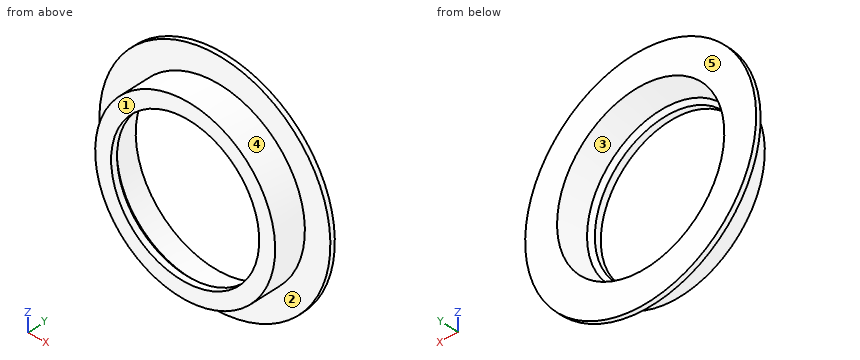
```python
from build123d import *

# Parameters (mm, degrees)
CHAMFER1_SIZE2 = 1
CHAMFER1_SIZE  = 1.294432523


with BuildPart() as part:
    # Sketch2 → Revolve1 (revolve)
    with BuildSketch(Plane.XY, mode=Mode.PRIVATE) as revolve1_sk:
        Polygon((28.25, 0), (28.25, 10), (36.25, 10), (36.25, 11.5), (26.25, 11.5), (24.25, 2), (23.25, 2), (23.25, 0), align=None)
    revolve(revolve1_sk.sketch.rotate(Axis((0, 0, 0), (0, 1, 0)), 90), axis=Axis((0, 0, 0), (0, 1, 0)))

    # Chamfer1
    chamfer1_edges = [part.edges().sort_by_distance(p)[0] for p in [
        (0, 2, 24.25),
    ]]
    chamfer1_side = [part.faces().sort_by_distance(p)[0] for p in [
        (0, 2.019570996, 24.25412021),
    ]]
    chamfer(chamfer1_edges, length=CHAMFER1_SIZE - 0.0001, length2=CHAMFER1_SIZE2 - 0.0001, reference=chamfer1_side[0])  # a hair under: the kernel refuses the full size


solid = part.part
```
For this review, take the finished solid that the model builds, in its own axes (mm). Face numbers are marked on the shaded views. A direction names the side the tool comes from. Coordinates: 2 decimals unless noted, no trailing zeros. Write each loop counter-clockwise with the first axis right and the second up, starting at its lowest first coordinate (ties: lowest second). Pieces come first, ordered by that corner, then holes. Notation, with made-up numbers: (79, -32.75) -> (99, -32.75) arc R12 cw to (99, -18.75) -> close; hole circle Ø10 at (81, 66). An arc over 180 degrees is marked (long way). Put each result on its own line as item: value.
Q1. Take a section at D-D, the plane y = 7. State the section outline as (x, z) points, then the cut area to 3 significant figures.
From the geometry:
outline: circle Ø56.5 at (0, 0); hole circle Ø50.61 at (0, 0)
area: 496 mm2
Q2. Clearance check with flat-ended pins moving along their axes: pin 1 Ø6 at (y, z) = (9, 11.5) entering from -X; pin 2 Ø4 at (x, y) = (-23.5, 9) entering from +Z; pin 3 Ø1.5 at (x, y) = (-22.5, 1.5) entering from -Z. State where each tip first meets the part, or that it passes through.
From the geometry:
pin 1: stops at x = -35.2
pin 2: stops at z = 28.99
pin 3: stops at z = -18.03
Q3. Tool access review of the marked faces 1 and 2: name each direction out of +Z, -Z, +X, -X, +Y, -Y from which nothing blocks a thin tool from reaching the whole face with its end or side.
From the geometry:
face 1: +Z, -Z, +X, -X, -Y
face 2: -Y
Q4. Wall thickness on L1, parallel to X at y = 1.4, z = 0; L2, parallel to Y at x = -7, z = -31; L3, parallel to X at y = 6, z = 1: over which ranges is each line inside the solid? List them lowest first.
From the geometry:
L1: x = -28.25 to -23.25, 23.25 to 28.25
L2: y = 10 to 11.5
L3: x = -28.23 to -25.07, 25.07 to 28.23
Q5. Take a section at C-C, the plane y = 1. State the section outline as (x, z) points.
From the geometry:
outline: circle Ø56.5 at (0, 0); hole circle Ø46.5 at (0, 0)
Q6. The part is to be moulded in two halves that separate along Z. For the marked faces 3, 4 and 5, say which applies: +Z half, -Z half, draft (parallel to the pull), parting line (faces both ways), or undercut.
From the geometry:
face 3: undercut
face 4: parting line
face 5: draft
